Design review of the part built by this model. Coordinates are the model's own, in mm. A direction names the side the tool comes from. Coordinates: 2 decimals unless noted, no trailing zeros. Loops run counter-clockwise (first coordinate to the right, second up) from the corner with the lowest first, then second, coordinate; pieces in that order, holes last. Notation, with made-up numbers: M 81.5,81 L 135.5,81 A13 cw 135.5,103 Z; hole C 74.25,54.25 d6. An arc over 180 degrees is marked long. Put each result on its own line as item: value. Start each with the question number.
(1) Take a section at C-C, the plane z = 585. Count the separate pieces of the cut face and the enclosed holes in it, then the cut area to 3 significant figures.
(2) Take a section at A-A, the plane x = 0. Give the boundary of the cut face in (y, z), then the cut area to 3 significant figures.
(3) The part is to be moulded in two halves that separate along Y. For faces 3 (the flat face through (-28.575, 762, 584)), 4 (the flat face through (-11, 778.631, 584)), 5 (the cylindrical face through (0.564, 787.523, 584.273)), say which applies: +Y half, -Y half, draft (parallel to the pull), parting line (faces both ways), or undercut.
(4) Take a section at B-B, the plane y = 739.5. Give the boundary of the cut face in (x, z).
(5) Clearance check with flat-ended pins moving along their axes: pin 1 (3 mm diameter, centred on x = 22.22, y = 740.53, fed in from -Z); pin 2 (4 mm diameter, centred on x = -11.5, z = 584.5, fed in from +Y). State where each tip first meets the part, or that it passes through.
(6) For faces 1 (the flat face through (0, 770, 589.102)), 2 (the flat face through (11, 778.631, 584)), list the 3-axis set-ups (+Z, -Z, +X, -X, +Y, -Y) from which the entire face can be reached by the end or side of a thin tool; tool diameter is ignored.
(7) For probe 1 along Y at (x, z) = (0, 582.25); probe 2 along Y at (x, z) = (23, 584.75); probe 3 along X at (y, z) = (787, 580.5), list the stretches that pass through material, from the lowest coordinate up. Write a range as [from, to].
```python
from build123d import *

# Parameters (mm, degrees)
SKETCH1_W           = 57.15
SKETCH1_H           = 57.15
SKETCH1_R           = 2.6035
SKETCH1_R_2         = 6.35
SKETCH1_R_3         = 1.5875
BOSS_EXTRUDE1_DEPTH = 9.525
CHAMFER1_SIZE       = 1.5875
FILLET1_R           = 6.35
SKETCH2_R           = 2.6035
CUT_EXTRUDE1_DEPTH  = 12.7


with BuildPart() as part:
    # Sketch1 → Boss-Extrude1 (new body)
    with BuildSketch(Plane.XY.offset(579.576994876)):
        with Locations((0, 762.756140976)):
            Rectangle(SKETCH1_W, SKETCH1_H)
        with Locations(Location((-22.225, 784.981140976, 0), (0, 0, 180))):
            Circle(SKETCH1_R, mode=Mode.SUBTRACT)
        with Locations(Location((0, 762.756140976, 0), (0, 0, 180))):
            Circle(SKETCH1_R_2, mode=Mode.SUBTRACT)
        with Locations(Location((-10.31875, 762.756140976, 0), (0, 0, 180))):
            Circle(SKETCH1_R_3, mode=Mode.SUBTRACT)
        with Locations(Location((10.31875, 762.756140976, 0), (0, 0, 180))):
            Circle(SKETCH1_R_3, mode=Mode.SUBTRACT)
        with Locations(Location((22.225, 784.981140976, 0), (0, 0, 180))):
            Circle(SKETCH1_R, mode=Mode.SUBTRACT)
        with Locations(Location((22.225, 762.756140976, 0), (0, 0, 180))):
            Circle(SKETCH1_R, mode=Mode.SUBTRACT)
        with Locations(Location((0, 784.981140976, 0), (0, 0, 180))):
            Circle(SKETCH1_R, mode=Mode.SUBTRACT)
        with Locations(Location((-22.225, 762.756140976, 0), (0, 0, 180))):
            Circle(SKETCH1_R, mode=Mode.SUBTRACT)
        with Locations(Location((22.225, 740.531140976, 0), (0, 0, 180))):
            Circle(SKETCH1_R, mode=Mode.SUBTRACT)
        with Locations(Location((0, 740.531140976, 0), (0, 0, 180))):
            Circle(SKETCH1_R, mode=Mode.SUBTRACT)
        with Locations(Location((-22.225, 740.531140976, 0), (0, 0, 180))):
            Circle(SKETCH1_R, mode=Mode.SUBTRACT)
    extrude(amount=BOSS_EXTRUDE1_DEPTH)

    # Chamfer1
    chamfer1_edges = [part.edges().sort_by_distance(p)[0] for p in [
        (-8.73125, 762.756140976, 589.101994876),
        (11.90625, 762.756140976, 589.101994876),
    ]]
    chamfer(chamfer1_edges, length=CHAMFER1_SIZE)

    # Fillet1
    fillet1_edges = [part.edges().sort_by_distance(p)[0] for p in [
        (28.575, 734.181140976, 584.339494876),
        (-28.575, 734.181140976, 584.339494876),
        (-28.575, 791.331140976, 584.339494876),
        (28.575, 791.331140976, 584.339494876),
    ]]
    fillet(fillet1_edges, radius=FILLET1_R)

    # Sketch2 → Cut-Extrude1 (cut)
    with BuildSketch(Plane(origin=(0, 791.331140976, 0), x_dir=(1, 0, 0), z_dir=(0, 1, 0))):
        with Locations(Location((-11.1125, -584.339494876, 0), (0, 0, 270))):
            Circle(SKETCH2_R)
        with Locations(Location((11.1125, -584.339494876, 0), (0, 0, 90))):
            Circle(SKETCH2_R)
    extrude(amount=-CUT_EXTRUDE1_DEPTH, mode=Mode.SUBTRACT)


solid = part.part
```
Computed values:
1. separate pieces: 1
1. enclosed holes: 11
1. area: 2,790 mm^2
2. outline: M 734.18,579.58 L 737.93,579.58 L 737.93,589.1 L 734.18,589.1 Z; M 743.13,579.58 L 756.41,579.58 L 756.41,589.1 L 743.13,589.1 Z; M 769.11,579.58 L 782.38,579.58 L 782.38,589.1 L 769.11,589.1 Z; M 787.58,579.58 L 791.33,579.58 L 791.33,589.1 L 787.58,589.1 Z
2. area: 324 mm^2
3. face 3: draft
3. face 4: +Y half
3. face 5: undercut
4. outline: M -28.49,579.58 L -24.62,579.58 L -24.62,589.1 L -28.49,589.1 Z; M -19.83,579.58 L -2.39,579.58 L -2.39,589.1 L -19.83,589.1 Z; M 2.39,579.58 L 19.83,579.58 L 19.83,589.1 L 2.39,589.1 Z; M 24.62,579.58 L 28.49,579.58 L 28.49,589.1 L 24.62,589.1 Z
5. pin 1: passes through
5. pin 2: stops at y = 778.63
6. face 1: +Z, +X, -X, +Y, -Y
6. face 2: +Y
7. probe 1: y = [734.18, 737.93], [743.13, 756.41], [769.11, 782.38], [787.58, 791.33]
7. probe 2: y = [734.23, 738.05], [743.02, 760.27], [765.24, 782.5], [787.47, 791.28]
7. probe 3: x = [-28.25, -23.87], [-20.58, -1.64], [1.64, 20.58], [23.87, 28.25]
